Model file for the job. Use its own axes, mm. A direction names the side the tool comes from. Round coordinates to 2 decimals unless told otherwise and drop trailing zeros. Loops run counter-clockwise (first coordinate to the right, second up) from the corner with the lowest first, then second, coordinate; pieces in that order, holes last. Notation, with made-up numbers: (57, 8.25) - (75, 8.25) arc R18 ccw to (75, 15.25) - close; hole circle Ø6 at (63.5, 51.25). An arc over 180 degrees is marked (long way). Answer as a JSON object with one key per item and string values.
from build123d import *

# Parameters (mm, degrees)
F0_R     = 100
F0_R_2   = 95
F0_R_3   = 80
F0_R_4   = 20
F1_DEPTH = 20
F2_R     = 80
F2_R_2   = 20
F3_DEPTH = 3
F4_R     = 80.0102
F4_R_2   = 20
F5_DEPTH = 3


with BuildPart() as f1:
    # F0 (on Top) → F1 (new body)
    with BuildSketch(Plane.XY):
        Circle(F0_R)
        Circle(F0_R_2, mode=Mode.SUBTRACT)
        Circle(F0_R_2)
        Circle(F0_R_3, mode=Mode.SUBTRACT)
        Circle(F0_R_3)
        Circle(F0_R_4, mode=Mode.SUBTRACT)
    extrude(amount=F1_DEPTH)

    # F2 (on face) → F3 (cut)
    with BuildSketch(Plane.XY.offset(20)):
        Circle(F2_R)
        Circle(F2_R_2, mode=Mode.SUBTRACT)
    extrude(amount=-F3_DEPTH, mode=Mode.SUBTRACT)

    # F4 (on face) → F5 (cut)
    with BuildSketch(Plane(origin=(0, 0, 0), x_dir=(1, 0, 0), z_dir=(0, 0, -1))):
        Circle(F4_R)
        Circle(F4_R_2, mode=Mode.SUBTRACT)
    extrude(amount=-F5_DEPTH, mode=Mode.SUBTRACT)


solid = f1.part
1) Two-plate mould, pull along X, no slides. Class faces 1 (the cylindrical face through (-17.34, -78.1, 18.52)), 2 (the flat face through (-45, 67, 0)), 3 (the cylindrical face through (95.38, 30.04, 9.86)): pulls with the +X half, pulls with the -X half, needs draft (parallel to the pull), parting line crosses it, or undercut.
Values follow:
{"face 1": "undercut", "face 2": "needs draft", "face 3": "parting line crosses it"}
2) Slice it at A-A on y = 0. List the corners of the cut face in (x, z), then the cut area to 3 significant figures.
Values follow:
{"outline": "(-100, 0) - (-80.01, 0) - (-80.01, 3) - (-20, 3) - (-20, 17) - (-80, 17) - (-80, 20) - (-100, 20) - close; (20, 3) - (80.01, 3) - (80.01, 0) - (100, 0) - (100, 20) - (80, 20) - (80, 17) - (20, 17) - close", "area": "2,480 mm²"}
3) Probe probe 1 along Y at (x, z) = (0, 18); probe 2 along Y at (x, z) = (0, 10.5); probe 3 along Z at (x, y) = (-45, -31). List the from-to ranges inside material, lowest first.
Values follow:
{"probe 1": "-100 to -80, 80 to 100", "probe 2": "-100 to -20, 20 to 100", "probe 3": "3 to 17"}
4) Tool access for faces 4 (the flat face through (-45, 67, 20)), 5 (the cylindrical face through (-63.493, 48.685, 1.479)), 6 (the flat face through (17, -17, 17)): list every direction of +Z, -Z, +X, -X, +Y, -Y with a clear straight run to the whole face (end or side of a thin tool).
Values follow:
{"face 4": "+Z, +X, -X, +Y, -Y", "face 5": "-Z", "face 6": "+Z"}
5) Slice it at C-C on z = 14. List the corners of the cut face in (x, y).
Values follow:
{"outline": "circle Ø200 at (0, 0); hole circle Ø40 at (0, 0)"}
6) Drop flat-ended pins along their axis: P1, Ø1.5, axis at x = 17, y = -13.5, coming from the +Z side; P2, Ø12, axis at x = 29.5, y = 20, coming from the -Z side; P3, Ø5, axis at x = 75, z = 15, coming from the -Y side. Give the stop position or say it passes through.
Values follow:
{"P1": "z = 17", "P2": "z = 3", "P3": "y = -68.87"}
7) Slice it at D-D on x = 49. List the corners of the cut face in (y, z), then the cut area to 3 significant figures.
Values follow:
{"outline": "(-87.17, 0) - (-63.25, 0) - (-63.25, 3) - (63.25, 3) - (63.25, 0) - (87.17, 0) - (87.17, 20) - (63.24, 20) - (63.24, 17) - (-63.24, 17) - (-63.24, 20) - (-87.17, 20) - close", "area": "2,730 mm²"}
